Build history of the part. All positions in model axes, mm. A direction names the side the tool comes from. Give positions to 0.01 mm unless a question says otherwise; leave off trailing zeros. Loops run counter-clockwise (first coordinate to the right, second up) from the corner with the lowest first, then second, coordinate; pieces in that order, holes last.
1) Flat gauge pins, fed straight in: P1, Ø5, axis at y = 266, z = -244.5, coming from the +X side; P2, Ø4, axis at x = 91.5, z = 129.5, coming from the +Y side; P3, Ø5, axis at x = 204.5, z = 54, coming from the +Y side. Where does each tip first touch, or does it go through?
2) Wall check: line 1 (Z direction, x = -16, y = 121); line 2 (X direction, y = 238.5, z = -199.5); line 3 (Y direction, x = 104.5, z = -236.3). Give the ranges that are in metal, low to high.
3) Band-saw the part on B-B on z = -207. List the corners of the cut face in (x, y).
4) Two-plate mould, pull along Y, no slides. Class faces 1 (the flat face through (150, 101, 328)), 2 (the flat face through (3, 0, 58)), 3 (the cylindrical face through (199.014, 138.708, 247.599)): +Y half, -Y half, draft (parallel to the pull), parting line (faces both ways), or undercut.
5) Band-saw the part on A-A on x = 88. List the corners of the cut face in (y, z), then the cut area to 3 significant figures.
6) 3-axis set-ups, long thin cutter, end or side, ignore diameter. For faces 4 (the flat face through (198, 140, 31)), 5 (the flat face through (149.081, 171.234, 320.121)), 6 (the cylindrical face through (-199.014, 225.358, -45.994)), 7 (the flat face through (175, 101, 292.174)): which of +Z, -Z, +X, -X, +Y, -Y reach the whole face in a straight line?
```python
from build123d import *

# Parameters (mm, degrees)
BOSS_EXTRUDE1_DEPTH     = 1.5
BOSS_EXTRUDE2_DEPTH     = 280
SKETCH4_W               = 400
SKETCH4_H               = 42.385541564
BOSS_EXTRUDE3_DEPTH     = 2
CUT_EXTRUDE1_DEPTH      = 609.61485268
CUT_EXTRUDE1_DEPTH_BACK = 609.61485268
SKETCH10_R              = 3
CUT_EXTRUDE2_DEPTH      = 2
SKETCH5_R               = 2
SKETCH5_R_2             = 10
CUT_EXTRUDE7_DEPTH      = 2
SKETCH21_W              = 300
SKETCH21_H              = 1.5
BOSS_EXTRUDE9_DEPTH     = 10
SKETCH22_W              = 300
SKETCH22_H              = 1.5
BOSS_EXTRUDE10_DEPTH    = 10
BOSS_EXTRUDE11_DEPTH    = 0.75
BOSS_EXTRUDE12_DEPTH    = 0.75
BOSS_EXTRUDE13_DEPTH    = 0.75
BOSS_EXTRUDE14_DEPTH    = 0.75
SKETCH27_W              = 200
SKETCH27_H              = 1.5
BOSS_EXTRUDE15_DEPTH    = 10
BOSS_EXTRUDE16_DEPTH    = 0.75
BOSS_EXTRUDE17_DEPTH    = 0.75
SKETCH30_R              = 24
SKETCH30_R_2            = 1.5
CUT_EXTRUDE8_DEPTH      = 2
SKETCH33_R              = 2
CUT_EXTRUDE9_DEPTH      = 2
SKETCH42_W              = 340
SKETCH42_H              = 12
SKETCH42_R              = 1.6
CUT_EXTRUDE13_DEPTH     = 40


with BuildPart() as part:
    # Sketch1 → Boss-Extrude1 (new body)
    with BuildSketch(Plane(origin=(0, 0, 0), x_dir=(1, 0, 0), z_dir=(0, 1, 0))):
        Polygon((-200, 237.826300096), (200, 237.826300096), (200, -292.173699904), (150, -292.173699904), (150, -362.173699904), (-200, -362.173699904), align=None)
    extrude(amount=BOSS_EXTRUDE1_DEPTH)

    # Sketch2 → Boss-Extrude2 (add)
    with BuildSketch(Plane(origin=(0, 1.5, 0), x_dir=(1, 0, 0), z_dir=(0, 1, 0))):
        Polygon((-200, 237.826300096), (-200, -362.173699904), (150, -362.173699904), (150, -292.173699904), (200, -292.173699904), (200, 237.826300096), align=None)
        Polygon((-198, 235.826300096), (-198, -360.173699904), (148, -360.173699904), (148, -290.173699904), (198, -290.173699904), (198, 235.826300096), align=None, mode=Mode.SUBTRACT)
    extrude(amount=BOSS_EXTRUDE2_DEPTH)

    # Sketch4 → Boss-Extrude3 (add)
    with BuildSketch(Plane(origin=(0, 0, -237.826300096), x_dir=(-1, 0, 0), z_dir=(0, 0, -1))):
        with Locations((0, 213.483316708)):
            Rectangle(SKETCH4_W, SKETCH4_H)
    extrude(amount=-BOSS_EXTRUDE3_DEPTH)

    # Sketch3 → Cut-Extrude1 (cut, two sides: drawn at the far end of the back side and taken through both)
    with BuildSketch(Plane.ZY.offset(200).offset(-CUT_EXTRUDE1_DEPTH_BACK)):
        Polygon((362.173699904, 121.117558148), (227.596852099, 281.5), (362.173699904, 281.5), align=None)
    extrude(amount=CUT_EXTRUDE1_DEPTH + CUT_EXTRUDE1_DEPTH_BACK, mode=Mode.SUBTRACT)

    # Sketch10 → Cut-Extrude2 (cut)
    with BuildSketch(Plane.ZY.offset(-148)):
        with BuildLine():
            Line((333.923699904, 90.5), (319.923699904, 90.5))
            Line((319.923699904, 90.5), (319.923699904, 87.5))
            Line((319.923699904, 87.5), (315.673699904, 87.5))
            ThreePointArc((315.673699904, 87.5), (304.673699904, 76.5), (315.673699904, 65.5))
            Line((315.673699904, 65.5), (338.173699904, 65.5))
            ThreePointArc((338.173699904, 65.5), (349.173699904, 76.5), (338.173699904, 87.5))
            Line((338.173699904, 87.5), (333.923699904, 87.5))
            Line((333.923699904, 87.5), (333.923699904, 90.5))
        make_face()
        with Locations((300.973699904, 103.45)):
            Circle(SKETCH10_R)
        with Locations((352.873699904, 103.45)):
            Circle(SKETCH10_R)
        with Locations((300.973699904, 49.55)):
            Circle(SKETCH10_R)
        with Locations((352.873699904, 49.55)):
            Circle(SKETCH10_R)
    extrude(amount=-CUT_EXTRUDE2_DEPTH, mode=Mode.SUBTRACT)

    # Sketch5 → Cut-Extrude7 (cut)
    with BuildSketch(Plane.ZY.offset(200)):
        with Locations((-115.826300096, 247.120648807)):
            Circle(SKETCH5_R)
        with Locations((-116.326300096, 223.125857706)):
            Circle(SKETCH5_R)
        with Locations((-91.826300096, 223.120648807)):
            Circle(SKETCH5_R)
        with Locations((-91.826300096, 247.120648807)):
            Circle(SKETCH5_R)
        with Locations((-103.826300096, 235.120648807)):
            Circle(SKETCH5_R_2)
        with Locations((-55.826300096, 247.120648807)):
            Circle(SKETCH5_R)
        with Locations((-56.326300096, 223.125857706)):
            Circle(SKETCH5_R)
        with Locations((-31.826300096, 223.120648807)):
            Circle(SKETCH5_R)
        with Locations((-31.826300096, 247.120648807)):
            Circle(SKETCH5_R)
        with Locations((-43.826300096, 235.120648807)):
            Circle(SKETCH5_R_2)
        with Locations((4.173699904, 247.120648807)):
            Circle(SKETCH5_R)
        with Locations((3.673699904, 223.125857706)):
            Circle(SKETCH5_R)
        with Locations((28.173699904, 223.120648807)):
            Circle(SKETCH5_R)
        with Locations((28.173699904, 247.120648807)):
            Circle(SKETCH5_R)
        with Locations((16.173699904, 235.120648807)):
            Circle(SKETCH5_R_2)
        with Locations((64.173699904, 247.120648807)):
            Circle(SKETCH5_R)
        with Locations((63.673699904, 223.125857706)):
            Circle(SKETCH5_R)
        with Locations((88.173699904, 223.120648807)):
            Circle(SKETCH5_R)
        with Locations((88.173699904, 247.120648807)):
            Circle(SKETCH5_R)
        with Locations((76.173699904, 235.120648807)):
            Circle(SKETCH5_R_2)
    extrude(amount=-CUT_EXTRUDE7_DEPTH, mode=Mode.SUBTRACT)

    # Sketch21 → Boss-Extrude9 (add)
    with BuildSketch(Plane(origin=(0, 0, -237.826300096), x_dir=(-1, 0, 0), z_dir=(0, 0, -1))):
        with Locations((0, 270.75)):
            Rectangle(SKETCH21_W, SKETCH21_H)
    extrude(amount=BOSS_EXTRUDE9_DEPTH)

    # Sketch22 → Boss-Extrude10 (add)
    with BuildSketch(Plane.ZY.offset(200)):
        with Locations((-7.826300096, 270.75)):
            Rectangle(SKETCH22_W, SKETCH22_H)
    boss_extrude10 = extrude(amount=BOSS_EXTRUDE10_DEPTH)

    # Sketch23 → Boss-Extrude11 (add, symmetric)
    with BuildSketch(Plane(origin=(0, 0, -77.826300096), x_dir=(-1, 0, 0), z_dir=(0, 0, -1))):
        Polygon((210, 270), (200, 270), (200, 260), align=None)
    boss_extrude11 = extrude(amount=BOSS_EXTRUDE11_DEPTH, both=True)

    # Sketch24 → Boss-Extrude12 (add, symmetric)
    with BuildSketch(Plane.XY.offset(52.173699904)):
        Polygon((-210, 270), (-200, 260), (-200, 270), align=None)
    boss_extrude12 = extrude(amount=BOSS_EXTRUDE12_DEPTH, both=True)

    # Sketch25 → Boss-Extrude13 (add, symmetric)
    with BuildSketch(Plane(origin=(100, 0, 0), x_dir=(0, 0, -1), z_dir=(1, 0, 0))):
        Polygon((247.826300096, 270), (237.826300096, 270), (237.826300096, 260), align=None)
    extrude(amount=BOSS_EXTRUDE13_DEPTH, both=True)

    # Sketch26 → Boss-Extrude14 (add, symmetric)
    with BuildSketch(Plane.ZY.offset(100)):
        Polygon((-247.826300096, 270), (-237.826300096, 260), (-237.826300096, 270), align=None)
    extrude(amount=BOSS_EXTRUDE14_DEPTH, both=True)

    # Mirror1: Boss-Extrude10, Boss-Extrude11, Boss-Extrude12 across plane
    add(boss_extrude10.mirror(Plane(origin=(0, 0, 0), x_dir=(0, 0, 1), z_dir=(1, 0, 0))))
    add(boss_extrude11.mirror(Plane(origin=(0, 0, 0), x_dir=(0, 0, 1), z_dir=(1, 0, 0))))
    add(boss_extrude12.mirror(Plane(origin=(0, 0, 0), x_dir=(0, 0, 1), z_dir=(1, 0, 0))))

    # Sketch27 → Boss-Extrude15 (add)
    with BuildSketch(Plane.XY.offset(362.173699904)):
        with Locations((-25, 110.367558148)):
            Rectangle(SKETCH27_W, SKETCH27_H)
    extrude(amount=BOSS_EXTRUDE15_DEPTH)

    # Sketch28 → Boss-Extrude16 (add, symmetric)
    with BuildSketch(Plane.ZY.offset(95)):
        Polygon((372.173699904, 109.617558148), (362.173699904, 109.617558148), (362.173699904, 99.617558148), align=None)
    extrude(amount=BOSS_EXTRUDE16_DEPTH, both=True)

    # Sketch29 → Boss-Extrude17 (add, symmetric)
    with BuildSketch(Plane(origin=(45, 0, 0), x_dir=(0, 0, -1), z_dir=(1, 0, 0))):
        Polygon((-372.173699904, 109.617558148), (-362.173699904, 99.617558148), (-362.173699904, 109.617558148), align=None)
    extrude(amount=BOSS_EXTRUDE17_DEPTH, both=True)

    # Sketch30 → Cut-Extrude8 (cut)
    with BuildSketch(Plane(origin=(200, 0, 0), x_dir=(0, 0, -1), z_dir=(1, 0, 0))):
        with Locations((-258.673699904, 160)):
            Circle(SKETCH30_R)
        with Locations((-284.673699904, 150)):
            Circle(SKETCH30_R_2)
        with Locations((-232.673699904, 150)):
            Circle(SKETCH30_R_2)
    extrude(amount=-CUT_EXTRUDE8_DEPTH, mode=Mode.SUBTRACT)

    # Sketch33 → Cut-Extrude9 (cut)
    with BuildSketch(Plane.ZY.offset(200)):
        with Locations((-180.626300096, 147.77)):
            Circle(SKETCH33_R)
        with Locations((-180.626300096, 28.39)):
            Circle(SKETCH33_R)
        with Locations((-8.926300096, 147.77)):
            Circle(SKETCH33_R)
        with Locations((-8.926300096, 28.39)):
            Circle(SKETCH33_R)
        with Locations((162.773699904, 147.77)):
            Circle(SKETCH33_R)
        with Locations((162.773699904, 28.39)):
            Circle(SKETCH33_R)
    extrude(amount=-CUT_EXTRUDE9_DEPTH, mode=Mode.SUBTRACT)

    # Sketch42 → Cut-Extrude13 (cut)
    with BuildSketch(Plane.XY.offset(-235.826300096)):
        with Locations((0, 225.5)):
            Rectangle(SKETCH42_W, SKETCH42_H)
        with Locations((-120.5, 240)):
            Circle(SKETCH42_R)
        with Locations((-149.5, 211)):
            Circle(SKETCH42_R)
        with Locations((-75.5, 240)):
            Circle(SKETCH42_R)
        with Locations((-104.5, 211)):
            Circle(SKETCH42_R)
        with Locations((-30.5, 240)):
            Circle(SKETCH42_R)
        with Locations((-59.5, 211)):
            Circle(SKETCH42_R)
        with Locations((14.5, 240)):
            Circle(SKETCH42_R)
        with Locations((-14.5, 211)):
            Circle(SKETCH42_R)
        with Locations((59.5, 240)):
            Circle(SKETCH42_R)
        with Locations((30.5, 211)):
            Circle(SKETCH42_R)
        with Locations((104.5, 240)):
            Circle(SKETCH42_R)
        with Locations((75.5, 211)):
            Circle(SKETCH42_R)
        with Locations((149.5, 240)):
            Circle(SKETCH42_R)
        with Locations((120.5, 211)):
            Circle(SKETCH42_R)
    extrude(amount=-CUT_EXTRUDE13_DEPTH, mode=Mode.SUBTRACT)


solid = part.part
```
Findings below:
1. P1: stops at x = 100.75
1. P2: stops at y = 1.5
1. P3: stops at y = 271.5
2. line 1: z = -237.83 to -235.83, 360.17 to 362.17
2. line 2: x = -200 to -198, 198 to 200
2. line 3: y = 0 to 219.5, 231.5 to 238.4, 241.6 to 281.5
3. outline: (-200, 0) - (200, 0) - (200, 281.5) - (198, 281.5) - (198, 1.5) - (-198, 1.5) - (-198, 281.5) - (-200, 281.5) - close
4. face 1: draft
4. face 2: -Y half
4. face 3: undercut
5. outline: (0, -237.83) - (219.5, -237.83) - (219.5, -235.83) - (1.5, -235.83) - (1.5, 360.17) - (123.5, 360.17) - (121.12, 362.17) - (0, 362.17) - close; (231.5, -237.83) - (270, -237.83) - (270, -247.83) - (271.5, -247.83) - (271.5, -237.83) - (281.5, -237.83) - (281.5, -235.83) - (231.5, -235.83) - close
5. area: 1,690 mm2
6. face 4: +Y
6. face 5: +Z, +X, -X, +Y
6. face 6: -X
6. face 7: +Z, +X, +Y, -Y
